from build123d import *

# Parameters (mm, degrees)
SKETCH1_W            = 50
SKETCH1_H            = 40
BOSS_EXTRUDE1_DEPTH  = 3
SKETCH6_R            = 2
CUT_EXTRUDE9_DEPTH   = 5
SKETCH16_W           = 14.8
SKETCH16_H           = 3
CUT_EXTRUDE10_DEPTH  = 0.5
SKETCH21_R           = 14.25
CUT_EXTRUDE15_DEPTH  = 4
CUT_EXTRUDE16_START  = -4
CUT_EXTRUDE16_DEPTH  = 4
SKETCH33_W           = 4
SKETCH33_H           = 35
CUT_EXTRUDE23_DEPTH  = 5
SKETCH34_W           = 49.986920535
SKETCH34_H           = 3
BOSS_EXTRUDE2_DEPTH  = 3
SKETCH35_W           = 50
SKETCH35_H           = 3
BOSS_EXTRUDE3_DEPTH  = 3
SKETCH36_W           = 46
SKETCH36_H           = 3
BOSS_EXTRUDE4_DEPTH  = 4
SKETCH38_W           = 3
SKETCH38_H           = 46
BOSS_EXTRUDE5_DEPTH  = 25
SKETCH39_W           = 45.535565308
SKETCH39_H           = 3
BOSS_EXTRUDE6_DEPTH  = 15
SKETCH40_W           = 46
SKETCH40_H           = 3
BOSS_EXTRUDE7_DEPTH  = 15
SKETCH41_W           = 0.464434692
SKETCH41_H           = 3
BOSS_EXTRUDE8_DEPTH  = 15
SKETCH42_R           = 2
CUT_EXTRUDE24_DEPTH  = 15
SKETCH43_R           = 2
CUT_EXTRUDE25_DEPTH  = 15
BOSS_EXTRUDE10_START = 1
SKETCH44_W           = 14.986920535
SKETCH44_H           = 46
SKETCH44_R           = 2
BOSS_EXTRUDE10_DEPTH = 1
BOSS_EXTRUDE11_START = 1
SKETCH46_W           = 15
SKETCH46_H           = 46
SKETCH46_R           = 2
BOSS_EXTRUDE11_DEPTH = 1
BOSS_EXTRUDE12_DEPTH = 2
BOSS_EXTRUDE13_DEPTH = 2
SKETCH49_W           = 47.986920535
SKETCH49_H           = 2
BOSS_EXTRUDE14_DEPTH = 10
CUT_EXTRUDE26_DEPTH  = 10


with BuildPart() as part:
    # Sketch1 → Boss-Extrude1 (new body)
    with BuildSketch(Plane(origin=(0, 0, 0), x_dir=(1, 0, 0), z_dir=(0, 1, 0))):
        with Locations((1.920937393, -5.615172506)):
            Rectangle(SKETCH1_W, SKETCH1_H)
    extrude(amount=BOSS_EXTRUDE1_DEPTH)

    # Sketch6 → Cut-Extrude9 (cut)
    with BuildSketch(Plane.XZ):
        with Locations(Location((6.920937393, 23.115172506, 0), (0, 0, 270))):
            Circle(SKETCH6_R)
        with Locations(Location((6.920937393, -11.884827494, 0), (0, 0, 270))):
            Circle(SKETCH6_R)
        with BuildLine():
            Line((24.420937393, 13.015172506), (18.923020545, 13.015172506))
            ThreePointArc((18.923020545, 13.015172506), (-7.179062607, 5.615172506), (18.923020545, -1.784827494))
            Line((18.923020545, -1.784827494), (24.420937393, -1.784827494))
            Line((24.420937393, -1.784827494), (24.420937393, 5.615172506))
            Line((24.420937393, 5.615172506), (24.420937393, 13.015172506))
        make_face()
    extrude(amount=-CUT_EXTRUDE9_DEPTH, mode=Mode.SUBTRACT)

    # Sketch16 → Cut-Extrude10 (cut)
    with BuildSketch(Plane.ZY.offset(-24.420937393)):
        with Locations((5.615172506, 1.5)):
            Rectangle(SKETCH16_W, SKETCH16_H)
    extrude(amount=-CUT_EXTRUDE10_DEPTH, mode=Mode.SUBTRACT)

    # Sketch21 → Cut-Extrude15 (cut)
    with BuildSketch(Plane(origin=(0, 0, 0), x_dir=(-1, 0, 0), z_dir=(0, -1, 0))):
        with Locations((-6.920937393, -5.615172506)):
            Circle(SKETCH21_R)
    extrude(amount=-CUT_EXTRUDE15_DEPTH, mode=Mode.SUBTRACT)

    # Sketch22 → Cut-Extrude16 (cut)
    with BuildSketch(Plane(origin=(0, 3, 0), x_dir=(1, 0, 0), z_dir=(0, 1, 0)).offset(CUT_EXTRUDE16_START)):
        with BuildLine():
            ThreePointArc((21.106680727, 1.784827494), (20.39103932, 3.019158274), (19.568281538, 4.184827494))
            Line((19.568281538, 4.184827494), (17.266105347, 4.184827494))
            ThreePointArc((17.266105347, 4.184827494), (18.246250908, 3.03351374), (19.09888878, 1.784827494))
            Line((19.09888878, 1.784827494), (21.106680727, 1.784827494))
        make_face()
        with BuildLine():
            Line((17.266105347, -15.415172506), (19.568281538, -15.415172506))
            ThreePointArc((19.568281538, -15.415172506), (20.39103932, -14.249503286), (21.106680727, -13.015172506))
            Line((21.106680727, -13.015172506), (19.09888878, -13.015172506))
            ThreePointArc((19.09888878, -13.015172506), (18.246250908, -14.263858752), (17.266105347, -15.415172506))
        make_face()
    extrude(amount=CUT_EXTRUDE16_DEPTH, mode=Mode.SUBTRACT)

    # Sketch33 → Cut-Extrude23 (cut)
    with BuildSketch(Plane(origin=(0, 3, 0), x_dir=(1, 0, 0), z_dir=(0, 1, 0))):
        with Locations((6.920937393, -5.615172506)):
            Rectangle(SKETCH33_W, SKETCH33_H)
    extrude(amount=-CUT_EXTRUDE23_DEPTH, mode=Mode.SUBTRACT)

    # Sketch34 → Boss-Extrude2 (add)
    with BuildSketch(Plane(origin=(0, 0, -14.384827494), x_dir=(-1, 0, 0), z_dir=(0, 0, -1))):
        with Locations((-1.927477126, 1.5)):
            Rectangle(SKETCH34_W, SKETCH34_H)
    extrude(amount=BOSS_EXTRUDE2_DEPTH)

    # Sketch35 → Boss-Extrude3 (add)
    with BuildSketch(Plane.XY.offset(25.615172506)):
        with Locations((1.920937393, 1.5)):
            Rectangle(SKETCH35_W, SKETCH35_H)
    extrude(amount=BOSS_EXTRUDE3_DEPTH)

    # Sketch36 → Boss-Extrude4 (add)
    with BuildSketch(Plane(origin=(26.920937393, 0, 0), x_dir=(0, 0, -1), z_dir=(1, 0, 0))):
        with Locations((-5.615172506, 1.5)):
            Rectangle(SKETCH36_W, SKETCH36_H)
    extrude(amount=BOSS_EXTRUDE4_DEPTH)

    # Sketch38 → Boss-Extrude5 (add)
    with BuildSketch(Plane(origin=(0, 3, 0), x_dir=(1, 0, 0), z_dir=(0, 1, 0))):
        with Locations((29.420937393, -5.615172506)):
            Rectangle(SKETCH38_W, SKETCH38_H)
        with Locations((-21.565983142, -5.615172506)):
            Rectangle(SKETCH38_W, SKETCH38_H)
    extrude(amount=BOSS_EXTRUDE5_DEPTH)

    # Sketch39 → Boss-Extrude6 (add)
    with BuildSketch(Plane.ZY.offset(23.065983142)):
        with Locations((5.38295516, 26.5)):
            Rectangle(SKETCH39_W, SKETCH39_H)
    extrude(amount=BOSS_EXTRUDE6_DEPTH)

    # Sketch40 → Boss-Extrude7 (add)
    with BuildSketch(Plane(origin=(30.920937393, 0, 0), x_dir=(0, 0, -1), z_dir=(1, 0, 0))):
        with Locations((-5.615172506, 26.5)):
            Rectangle(SKETCH40_W, SKETCH40_H)
    extrude(amount=BOSS_EXTRUDE7_DEPTH)

    # Sketch41 → Boss-Extrude8 (add)
    with BuildSketch(Plane.ZY.offset(23.065983142)):
        with Locations((28.38295516, 26.5)):
            Rectangle(SKETCH41_W, SKETCH41_H)
    extrude(amount=BOSS_EXTRUDE8_DEPTH)

    # Sketch42 → Cut-Extrude24 (cut)
    with BuildSketch(Plane.XZ.offset(-25)):
        with Locations(Location((38.420937393, 20.419520332, 0), (0, 0, 270))):
            Circle(SKETCH42_R)
        with Locations(Location((38.420937393, -8.692413747, 0), (0, 0, 270))):
            Circle(SKETCH42_R)
    extrude(amount=-CUT_EXTRUDE24_DEPTH, mode=Mode.SUBTRACT)

    # Sketch43 → Cut-Extrude25 (cut)
    with BuildSketch(Plane.XZ.offset(-25)):
        with Locations(Location((-30.565983142, 20.419520332, 0), (0, 0, 270))):
            Circle(SKETCH43_R)
        with Locations(Location((-30.565983142, -8.692413747, 0), (0, 0, 270))):
            Circle(SKETCH43_R)
    extrude(amount=-CUT_EXTRUDE25_DEPTH, mode=Mode.SUBTRACT)

    # Sketch44 → Boss-Extrude10 (add)
    with BuildSketch(Plane.XZ.offset(-25).offset(BOSS_EXTRUDE10_START)):
        with Locations((-30.572522875, 5.615172506)):
            Rectangle(SKETCH44_W, SKETCH44_H)
        with Locations(Location((-30.565983142, -8.692413747, 0), (0, 0, 270))):
            Circle(SKETCH44_R, mode=Mode.SUBTRACT)
        with Locations(Location((-30.565983142, 20.419520332, 0), (0, 0, 270))):
            Circle(SKETCH44_R, mode=Mode.SUBTRACT)
    extrude(amount=-BOSS_EXTRUDE10_DEPTH)

    # Sketch46 → Boss-Extrude11 (add)
    with BuildSketch(Plane.XZ.offset(-25).offset(BOSS_EXTRUDE11_START)):
        with Locations((38.420937393, 5.615172506)):
            Rectangle(SKETCH46_W, SKETCH46_H)
        with Locations(Location((38.420937393, -8.692413747, 0), (0, 0, 270))):
            Circle(SKETCH46_R, mode=Mode.SUBTRACT)
        with Locations(Location((38.420937393, 20.419520332, 0), (0, 0, 270))):
            Circle(SKETCH46_R, mode=Mode.SUBTRACT)
    extrude(amount=-BOSS_EXTRUDE11_DEPTH)

    # Sketch47 → Boss-Extrude12 (add)
    with BuildSketch(Plane(origin=(0, 0, -17.384827494), x_dir=(-1, 0, 0), z_dir=(0, 0, -1))):
        Polygon((-27.920937393, 28), (-45.920937393, 28), (-45.920937393, 24), (-30.920937393, 24), (-30.920937393, 0), (23.065983142, 0), (23.065983142, 3), (23.065983142, 25), (23.079062607, 25), (23.079062607, 24), (37.960253495, 24), (37.960253495, 28), (20.065983142, 28), (20.065983142, 3), (-27.920937393, 3), align=None)
    extrude(amount=BOSS_EXTRUDE12_DEPTH)

    # Sketch48 → Boss-Extrude13 (add)
    with BuildSketch(Plane.XY.offset(28.615172506)):
        Polygon((-20.065983142, 28), (-37.960253495, 28), (-37.960253495, 24), (-23.079062607, 24), (-23.079062607, 25), (-23.065983142, 25), (-23.065983142, 3), (-23.065983142, 0), (30.920937393, 0), (30.920937393, 24), (45.920937393, 24), (45.920937393, 28), (27.920937393, 28), (27.920937393, 3), (-20.065983142, 3), align=None)
    extrude(amount=BOSS_EXTRUDE13_DEPTH)

    # Sketch49 → Boss-Extrude14 (add)
    with BuildSketch(Plane(origin=(0, 3, 0), x_dir=(1, 0, 0), z_dir=(0, 1, 0))):
        with Locations((3.927477126, 18.384827494)):
            Rectangle(SKETCH49_W, SKETCH49_H)
    extrude(amount=BOSS_EXTRUDE14_DEPTH)

    # Sketch50 → Cut-Extrude26 (cut)
    with BuildSketch(Plane.XY.offset(-17.384827494)):
        Polygon((-20.065983142, 13), (-9.830586805, 2.764603663), (17.920937393, 3), (27.920937393, 13), align=None)
    extrude(amount=-CUT_EXTRUDE26_DEPTH, mode=Mode.SUBTRACT)


solid = part.part
Design review of the part built by this model. Coordinates are the model's own, in mm. A direction names the side the tool comes from. Round coordinates to 2 decimals unless told otherwise and drop trailing zeros. Write each loop counter-clockwise with the first axis right and the second up, starting at its lowest first coordinate (ties: lowest second). Pieces come first, ordered by that corner, then holes. Notation, with made-up numbers: (62, 44.5) -> (73, 44.5) arc R8 ccw to (73, 48.5) -> close; hole circle Ø11 at (-2.5, 14.25). An arc over 180 degrees is marked (long way). One line per item, written item: value. Start each with the question number.
Q1. Add section C-C (x = 0). Give the boundary of the cut face in (y, z), then the cut area to 3 significant figures.
Q2. Tool access review of faces 1 (the face through (22.85, 7.93, -18.37)), 2 (the face through (27.921, 16, 5)), 3 (the face through (45.921, 26, 5)), 4 (the face through (23, 1, 13.015)), 5 (the face through (-38.066, 26, 5)): name each direction out of +Z, -Z, +X, -X, +Y, -Y from which nothing blocks a thin tool from reaching the whole face with its end or side.
Q3. Add section A-A (y = 20.5). Give the boundary of the cut face in (x, z).
Q4. To check wall thickness, follow probe 1 along X at (y, z) = (25.75, 18); probe 2 along X at (y, z) = (13, 6); probe 3 along Y at (x, z) = (-32.5, 6.5). State the ranges of each line that lie inside material, in increasing order.
Q5. Insertion check: P1, Ø5, axis at x = -30.57, z = 20.42, coming from the +Y side; P2, Ø3, axis at y = 17.5, z = -11.5, coming from the -X side; P3, Ø6, axis at x = -8.5, y = 8.5, coming from the +Z side; P4, Ø8, axis at y = 7, z = 2, coming from the +X side. Each pin has a flat end and moves straight along its axis. Give the tip position at first contact, or say it passes through.
Q6. The part is to be moulded in two halves that separate along Z. For faces 6 (the face through (-31, 24, 5)), 7 (the face through (25, 6, -17.385)), 8 (the face through (8.921, 2, -10)), say which applies: pulls with the +Z half, pulls with the -Z half, needs draft (parallel to the pull), parting line crosses it, or undercut.
Response:
1. outline: (0, -19.38) -> (2.85, -19.38) -> (2.85, -17.38) -> (3, -17.38) -> (3, -6.84) -> (0, -6.84) -> close; (0, 18.07) -> (3, 18.07) -> (3, 30.62) -> (0, 30.62) -> close
1. area: 75.0 mm^2
2. face 1: +Z, -Z, +Y
2. face 2: +Z, +Y
2. face 3: +Z, -Z, +X, +Y, -Y
2. face 4: +Y, -Y
2. face 5: +Z, -Z, -X, +Y, -Y
3. outline: (-23.07, -19.38) -> (-20.07, -19.38) -> (-20.07, 30.62) -> (-23.07, 30.62) -> close; (27.92, -19.38) -> (30.92, -19.38) -> (30.92, 30.62) -> (27.92, 30.62) -> close
4. probe 1: x = -38.07 to -20.07, 27.92 to 45.92
4. probe 2: x = -23.07 to -20.07, 27.92 to 30.92
4. probe 3: y = 24 to 28
5. P1: stops at y = 28
5. P2: stops at x = -23.07
5. P3: passes through
5. P4: stops at x = 30.92
6. face 6: needs draft
6. face 7: pulls with the +Z half
6. face 8: undercut
